Read the model definition and answer for the solid it produces. Units are mm, in the model's axes. A direction names the side the tool comes from. Coordinates: 2 decimals unless noted, no trailing zeros. Order: outer loops, then holes, each group sorted by start corner. A loop starts at its lowest first (then second) coordinate and runs counter-clockwise, first axis right, second up. Notation, with made-up numbers: (31, -4.5) -> (52, -4.5) arc R27 cw to (52, 16.5) -> close; hole circle Ø6 at (42, -7.5). An arc over 180 degrees is marked (long way). Return JSON: item names as keys, results as strings. Group by question number.
```python
from build123d import *

# Parameters (mm, degrees)
SKETCH1_W           = 12.7
SKETCH1_H           = 25.4
SKETCH1_H_2         = 19.05
SKETCH1_R           = 3.175
BOSS_EXTRUDE1_DEPTH = 1.5875
SKETCH1_3_W         = 1.5875
SKETCH1_3_H         = 25.4
BOSS_EXTRUDE2_DEPTH = 25.4
SKETCH2_R           = 3.175
CUT_EXTRUDE1_DEPTH  = 44.649033494
FILLET1_R           = 12.7
FILLET2_R           = 6.35


with BuildPart() as part:
    # Sketch1 → Boss-Extrude1 (new body)
    # profile 1 of 2: a face of its own
    with BuildSketch(Plane.XY):
        Rectangle(SKETCH1_W, SKETCH1_H)
    # profile 2 of 2: a face of its own
    with BuildSketch(Plane.XY):
        with Locations((0, 22.225)):
            Rectangle(SKETCH1_W, SKETCH1_H_2)
        with Locations((0, 25.4)):
            Circle(SKETCH1_R, mode=Mode.SUBTRACT)
    extrude(amount=BOSS_EXTRUDE1_DEPTH)

    # Sketch1<3> → Boss-Extrude2 (add)
    with BuildSketch(Plane.XY):
        with Locations((-7.14375, 0)):
            Rectangle(SKETCH1_3_W, SKETCH1_3_H)
        with Locations((7.14375, 0)):
            Rectangle(SKETCH1_3_W, SKETCH1_3_H)
    extrude(amount=BOSS_EXTRUDE2_DEPTH)

    # Sketch2 → Cut-Extrude1 (cut, through all)
    with BuildSketch(Plane.ZY.offset(7.9375)):
        with Locations((12.7, 0)):
            Circle(SKETCH2_R)
    extrude(amount=-CUT_EXTRUDE1_DEPTH, mode=Mode.SUBTRACT)

    # Fillet1
    fillet1_edges = [part.edges().sort_by_distance(p)[0] for p in [
        (-7.14375, -12.7, 25.4),
        (7.14375, -12.7, 25.4),
        (7.14375, 12.7, 25.4),
        (-7.14375, 12.7, 25.4),
    ]]
    fillet(fillet1_edges, radius=FILLET1_R - 0.0001)  # a hair under: the kernel refuses the full size

    # Fillet2
    fillet2_edges = [part.edges().sort_by_distance(p)[0] for p in [
        (-6.35, 31.75, 0.79375),
        (6.35, 31.75, 0.79375),
    ]]
    fillet(fillet2_edges, radius=FILLET2_R - 0.0001)  # a hair under: the kernel refuses the full size


solid = part.part
```
1. Given pin 1 (0.8 mm diameter, centred on y = 20.5, z = 1, fed in from +X); pin 2 (1.5 mm diameter, centred on y = 20, z = 3, fed in from -X); pin 3 (0.8 mm diameter, centred on x = 7, z = 6.5, fed in from +Y); pin 4 (1.7 mm diameter, centred on y = 22, z = 1, fed in from -X), each flat-ended and moving along its own axis, determine where each tip first touches the part or whether it passes through.
2. Find section A-A on z = 6.25. Determine the outline of the cut face in (x, y), and give its area (3 significant figures).
3. Which of the six approach directions +Z, -Z, +X, -X, +Y, -Y give full straight-line access (tool end or side, diameter ignored) to faces 1 (the face through (-7.15, 0.14, 9.53)), 2 (the face through (-6.35, 19, 1)), 3 (the face through (-7.13, 8.88, 21.78)), 4 (the face through (-6.35, 3, 11)), 5 (the face through (6.35, 19, 1))?
4. Find section C-C on x = 2.25. Determine the outline of the cut face in (y, z), and give its area (3 significant figures).
5. Straight lines are drawn through the part: L1, parallel to Y at x = 7.5, z = 12.7 (3 decimals); L2, parallel to X at y = -4, z = 4.75; L3, parallel to Y at x = 0, z = 0.45 (3 decimals). For each, find the intervals that lie inside material, in ascending order.
6. Find section D-D on y = 12. Determine the outline of the cut face in (x, z).
7. Find section B-B on y = -1. Determine the outline of the cut face in (x, z), and give its area (3 significant figures).
8. For a pull along Y with two mould halves and no side action, classify faces 6 (the face through (7.15, 8.88, 21.78)), 7 (the face through (-7.13, -9.08, 21.58)), 8 (the face through (-0.41, 28.55, 0.78)) as released by +Y, released by -Y, zero draft, split by the parting line, or undercut.
Result:
{
 "1": {"pin 1": "x = 6.35", "pin 2": "through", "pin 3": "y = 12.7", "pin 4": "x = -6.35"},
 "2": {"outline": "(-7.94, -12.7) -> (-6.35, -12.7) -> (-6.35, 12.7) -> (-7.94, 12.7) -> close; (6.35, -12.7) -> (7.94, -12.7) -> (7.94, 12.7) -> (6.35, 12.7) -> close", "area": "80.6 mm^2"},
 "3": {"face 1": "+X, -X", "face 2": "+Z, -Z, -X, +Y", "face 3": "+Z, +X, -X, +Y", "face 4": "+Z, +Y, -Y", "face 5": "+Z, -Z, +X, +Y"},
 "4": {"outline": "(-12.7, 0) -> (23.16, 0) -> (23.16, 1.59) -> (-12.7, 1.59) -> close; (27.64, 0) -> (31.34, 0) -> (31.34, 1.59) -> (27.64, 1.59) -> close", "area": "62.8 mm^2"},
 "5": {"L1": "-12.7 to -3.175, 3.175 to 12.7", "L2": "-7.94 to -6.35, 6.35 to 7.94", "L3": "-12.7 to 22.225, 28.575 to 31.75"},
 "6": {"outline": "(-7.94, 0) -> (7.94, 0) -> (7.94, 16.86) -> (6.35, 16.86) -> (6.35, 1.59) -> (-6.35, 1.59) -> (-6.35, 16.86) -> (-7.94, 16.86) -> close"},
 "7": {"outline": "(-7.94, 0) -> (7.94, 0) -> (7.94, 9.69) -> (6.35, 9.69) -> (6.35, 1.59) -> (-6.35, 1.59) -> (-6.35, 9.69) -> (-7.94, 9.69) -> close; (-7.94, 15.71) -> (-6.35, 15.71) -> (-6.35, 25.36) -> (-7.94, 25.36) -> close; (6.35, 15.71) -> (7.94, 15.71) -> (7.94, 25.36) -> (6.35, 25.36) -> close", "area": "81.5 mm^2"},
 "8": {"face 6": "released by +Y", "face 7": "released by -Y", "face 8": "undercut"}
}
